from build123d import *

# Parameters (mm, degrees)
Y_KSEKLIK_EKSTR_ZYON1_DEPTH = 100
Y_KSEKLIK_EKSTR_ZYON2_DEPTH = 5
Y_KSEKLIK_EKSTR_ZYON2_DRAFT = 45
IZIM6_R                     = 34.5
Y_KSEKLIK_EKSTR_ZYON3_DEPTH = 5
IZIM7_R                     = 31
Y_KSEKLIK_EKSTR_ZYON4_DEPTH = 15
IZIM8_R                     = 2
KES_EKSTR_ZYON1_DEPTH       = 5
DAIRESEL_KAPLAMA1_COUNT     = 12
Y_KSEKLIK_EKSTR_ZYON5_DEPTH = 100
Y_KSEKLIK_EKSTR_ZYON6_START = 10
IZIM11_R                    = 31
Y_KSEKLIK_EKSTR_ZYON6_DEPTH = 10
IZIM12_R                    = 30
Y_KSEKLIK_EKSTR_ZYON7_DEPTH = 11
IZIM13_R                    = 42.5
Y_KSEKLIK_EKSTR_ZYON8_DEPTH = 10.5
Y_KSEKLIK_EKSTR_ZYON9_DEPTH = 55
IZIM17_R                    = 15
KES_EKSTR_ZYON2_DEPTH       = 20
IZIM18_R                    = 15
KES_EKSTR_ZYON3_DEPTH       = 20


# Read off the part's stored shape, not the designer's step: Yükseklik-Ekstrüzyon2
with BuildPart() as part:
    # Çizim1 → Yükseklik-Ekstrüzyon1 (new body)
    with BuildSketch(Plane(origin=(0, 0, 0), x_dir=(1, 0, 0), z_dir=(0, 1, 0))):
        with BuildLine():
            Line((-37.5, 45), (37.5, 45))
            ThreePointArc((37.5, 45), (45.880962103, 0), (37.5, -45))
            Line((37.5, -45), (-37.5, -45))
            ThreePointArc((-37.5, -45), (-45.880962103, 0), (-37.5, 45))
        make_face()
    extrude(amount=-Y_KSEKLIK_EKSTR_ZYON1_DEPTH)


with BuildPart() as y_kseklik_ekstr_zyon2_tool:
    # Yükseklik-Ekstrüzyon2 outline → Yükseklik-Ekstrüzyon2 (with draft: the straight prism first)
    with BuildSketch(Plane(origin=(0, 5, 0), x_dir=(1, 0, 0), z_dir=(0, 1, 0))):
        with BuildLine():
            ThreePointArc((-34.018047093, 40), (-40.880962103, 0), (-34.018047093, -40))
            Line((-34.018047093, -40), (34.018047093, -40))
            ThreePointArc((34.018047093, -40), (40.880962103, 0), (34.018047093, 40))
            Line((34.018047093, 40), (-34.018047093, 40))
        make_face()
    extrude(amount=-Y_KSEKLIK_EKSTR_ZYON2_DEPTH)
    # Yükseklik-Ekstrüzyon2: the draft: its side faces are tilted about the plane it starts from
    y_kseklik_ekstr_zyon2_sides = [y_kseklik_ekstr_zyon2_tool.faces().sort_by_distance(p)[0] for p in [
        (0, 2.5, -40),
        (-40.880962103, 2.5, 0),
        (0, 2.5, 40),
        (40.880962103, 2.5, 0),
    ]]
    draft(y_kseklik_ekstr_zyon2_sides, Plane(origin=(0, 5, 0), x_dir=(1, 0, 0), z_dir=(0, 1, 0)), Y_KSEKLIK_EKSTR_ZYON2_DRAFT)


with BuildPart() as part_1:
    add(part.part)

    # Yükseklik-Ekstrüzyon2: add y_kseklik_ekstr_zyon2_tool
    add(y_kseklik_ekstr_zyon2_tool.part)

    # Çizim6 → Yükseklik-Ekstrüzyon3 (add, symmetric)
    with BuildSketch(Plane(origin=(0, 5, 0), x_dir=(1, 0, 0), z_dir=(0, 1, 0))):
        with Locations(Location((0, 0, 0), (0, 0, 270))):
            Circle(IZIM6_R)
    extrude(amount=Y_KSEKLIK_EKSTR_ZYON3_DEPTH, both=True)

    # Çizim7 → Yükseklik-Ekstrüzyon4 (add, symmetric)
    with BuildSketch(Plane(origin=(0, 10, 0), x_dir=(1, 0, 0), z_dir=(0, 1, 0))):
        with Locations(Location((0, 0, 0), (0, 0, 270))):
            Circle(IZIM7_R)
    extrude(amount=Y_KSEKLIK_EKSTR_ZYON4_DEPTH, both=True)

    # Çizim8 → Kes-Ekstrüzyon1 (cut)
    with BuildSketch(Plane(origin=(0, 25, 0), x_dir=(1, 0, 0), z_dir=(0, 1, 0))):
        with Locations(Location((27, 0, 0), (0, 0, 270))):
            Circle(IZIM8_R)
    kes_ekstr_zyon1 = extrude(amount=-KES_EKSTR_ZYON1_DEPTH, mode=Mode.SUBTRACT)

    # Dairesel Kaplama1: Kes-Ekstrüzyon1 ×12 about axis
    dairesel_kaplama1_axis = Axis((0, 0, 0), (0, 1, 0))
    for i in range(1, DAIRESEL_KAPLAMA1_COUNT):
        add(kes_ekstr_zyon1.rotate(dairesel_kaplama1_axis, i * 360 / DAIRESEL_KAPLAMA1_COUNT), mode=Mode.SUBTRACT)

    # Çizim10 → Yükseklik-Ekstrüzyon5 (add)
    with BuildSketch(Plane(origin=(0, 25, 0), x_dir=(1, 0, 0), z_dir=(0, 1, 0))):
        with BuildLine():
            Line((-15.581702618, -15.971995333), (-15.581702618, 18.028004667))
            ThreePointArc((-15.581702618, 18.028004667), (0, 21.342270575), (15.581702618, 18.028004667))
            Line((15.581702618, 18.028004667), (15.581702618, -15.971995333))
            ThreePointArc((15.581702618, -15.971995333), (0, -19.28626124), (-15.581702618, -15.971995333))
        make_face()
    extrude(amount=Y_KSEKLIK_EKSTR_ZYON5_DEPTH)

    # Çizim11 → Yükseklik-Ekstrüzyon6 (add)
    with BuildSketch(Plane(origin=(0, 125, 0), x_dir=(1, 0, 0), z_dir=(0, 1, 0)).offset(Y_KSEKLIK_EKSTR_ZYON6_START)):
        with Locations(Location((0, 0, 0), (0, 0, 270))):
            Circle(IZIM11_R)
    extrude(amount=-Y_KSEKLIK_EKSTR_ZYON6_DEPTH)

    # Çizim12 → Yükseklik-Ekstrüzyon7 (add)
    with BuildSketch(Plane(origin=(0, 135, 0), x_dir=(1, 0, 0), z_dir=(0, 1, 0))):
        with Locations(Location((0, 0, 0), (0, 0, 270))):
            Circle(IZIM12_R)
    extrude(amount=Y_KSEKLIK_EKSTR_ZYON7_DEPTH)

    # Çizim13 → Yükseklik-Ekstrüzyon8 (add, symmetric)
    with BuildSketch(Plane.ZY.offset(37.5)):
        with Locations(Location((45, -50, 0), (0, 0, 270))):
            Circle(IZIM13_R)
    extrude(amount=Y_KSEKLIK_EKSTR_ZYON8_DEPTH, both=True)

    # Çizim16 → Yükseklik-Ekstrüzyon9 (add)
    with BuildSketch(Plane(origin=(-27, 0, 0), x_dir=(0, 0, -1), z_dir=(1, 0, 0))):
        with BuildLine():
            Line((-45, -30), (-45, -70))
            Line((-45, -70), (-75, -70))
            ThreePointArc((-75, -70), (-82.639320225, -50), (-75, -30))
            Line((-75, -30), (-45, -30))
        make_face()
    extrude(amount=Y_KSEKLIK_EKSTR_ZYON9_DEPTH)

    # Çizim17 → Kes-Ekstrüzyon2 (cut)
    with BuildSketch(Plane(origin=(0, 146, 0), x_dir=(1, 0, 0), z_dir=(0, 1, 0))):
        with Locations(Location((0, 0, 0), (0, 0, 270))):
            Circle(IZIM17_R)
    extrude(amount=-KES_EKSTR_ZYON2_DEPTH, mode=Mode.SUBTRACT)

    # Çizim18 → Kes-Ekstrüzyon3 (cut)
    with BuildSketch(Plane.ZY.offset(48)):
        with Locations(Location((45, -50, 0), (0, 0, 270))):
            Circle(IZIM18_R)
    extrude(amount=-KES_EKSTR_ZYON3_DEPTH, mode=Mode.SUBTRACT)


solid = part_1.part
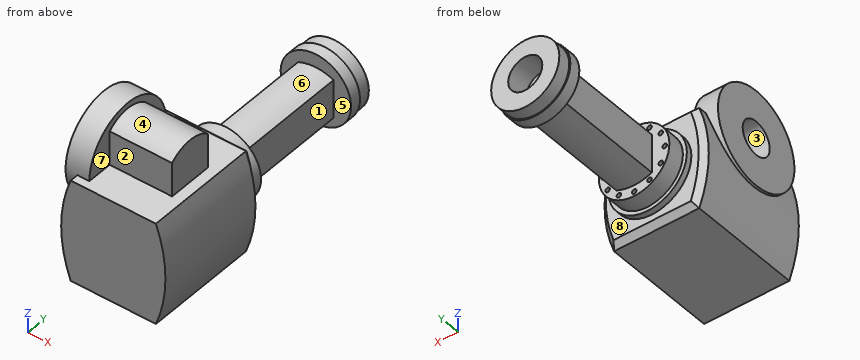
Input: part model. Units: mm. Frame: model coordinates. Face numbers are marked on the shaded views. A direction names the side the tool comes from. Give positions to 0.01 mm unless a question says otherwise; leave off trailing zeros. Loops run counter-clockwise (first coordinate to the right, second up) from the corner with the lowest first, then second, coordinate; pieces in that order, holes last. Notation, with made-up numbers: M 17.25,52 L 37.25,52 A10 ccw 37.25,65 Z; hole C -30,41 d2. An arc over 180 degrees is marked long. Use one line per item in the form item = value.
1. Section query A-A, the plane y = 55.5. Return the cut outline in (x, z).
Numbers:
outline = M -15.58,-18.03 A38.29 ccw 15.58,-18.03 L 15.58,15.97 A38.29 ccw -15.58,15.97 Z
2. Line query: L1, parallel to X at y = 22.3, z = 0; L2, parallel to Y at x = -19, z = 16; L3, parallel to X at y = 130.5, z = 0. Output: solid intervals per line, ascending.
Numbers:
L1 = -31 to -29, -25 to 25, 29 to 31
L2 = -100 to 25, 125 to 146
L3 = -31 to -15, 15 to 31
3. Reachability of the marked faces 1, 2, 3, 4 and 5 from +Z, -Z, +X, -X, +Y, -Y: full face, straight path, thin tool, end or side. Return the list, or none.
Numbers:
face_1 = +Z, -Z, +X
face_2 = +Z, +X, -Y
face_3 = -X
face_4 = +Z, +X
face_5 = none
4. Section query D-D, the plane y = -14.5. Return the cut outline in (x, z), and give its area (3 significant figures).
Numbers:
outline = M -48,21.63 L -43.99,21.63 A125 ccw -37.5,-45 L 37.5,-45 A125 ccw 37.5,45 L -27,45 L -27,68.37 L -48,68.37 Z
area = 8,410 mm²
5. Section query C-C, the plane y = -59. Return the cut outline in (x, z).
Numbers:
outline = M -48,3.46 L -45.83,3.46 A125 ccw -37.5,-45 L 37.5,-45 A125 ccw 37.5,45 L 28,45 L 28,81.26 L -27,81.26 L -27,86.54 L -48,86.54 L -48,57 L -28,57 L -28,33 L -48,33 Z
6. First-contact query: pin 1 (3 mm diameter, centred on y = -53.5, z = -17.5, fed in from +X); pin 2 (12 mm diameter, centred on y = 9, z = 37, fed in from -X); pin 3 (9 mm diameter, centred on x = -7, z = 3.5, fed in from +Y). Flat tips, straight axial feed; report the tip coordinate or a pass-through.
Numbers:
pin_1 = 44.85
pin_2 = -37.41
pin_3 = 126
7. Pull-direction query (Y, two-part tool) for the marked faces 6, 7 and 8; classes: released by +Y, released by -Y, zero draft, split by the parting line, or undercut.
Numbers:
face_6 = undercut
face_7 = zero draft
face_8 = released by +Y
